Input: part model. Units: mm. Frame: model coordinates. Face numbers are marked on the shaded views. A direction names the side the tool comes from. Round coordinates to 2 decimals unless told otherwise and drop trailing zeros. Loops run counter-clockwise (first coordinate to the right, second up) from the corner with the lowest first, then second, coordinate; pieces in that order, holes last. Notation, with made-up numbers: (31, 51.5) - (42, 51.5) arc R35 ccw to (42, 89.5) - close; hole circle Ø9 at (44, 39). An arc over 180 degrees is marked (long way). One line per question, with ' | ' between items. Start each with the question number.
Item 1: Section D-D, the plane y = -21.25. Return loops of the section in (x, z), plus the area to 3 significant figures.
Item 2: Section A-A, the plane x = 6.5. Return loops of the section in (y, z), plus the area to 3 significant figures.
Item 3: Section B-B, the plane y = -8.75. Return loops of the section in (x, z).
Item 4: Material intervals for line 1 along Y through (x, z) = (26.5, 7); line 2 along X through (y, z) = (-4.25, 8.5); line 3 along X through (y, z) = (-1.5, 26), sorted ascending.
Item 5: First-contact query: pin 1 (19 mm diameter, centred on x = 9.5, z = 25.5, fed in from -Y). Flat tip, straight axial feed; report the tip coordinate or a pass-through.
Item 6: Section C-C, the plane z = 10.5. Return loops of the section in (x, y).
Item 7: Set-up query: the marked faces 1 and 2. Return all of +Z, -Z, +X, -X, +Y, -Y with unobstructed straight access to the full face (end or side cutting, diameter ignored); none if empty.
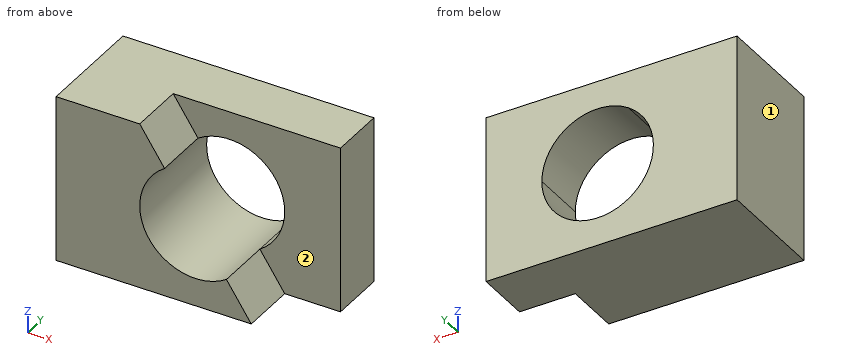
```python
from build123d import *

# Parameters (mm, degrees)
F0_W     = 57.15
F0_H     = 38.1
F1_DEPTH = 25.4
F2_W     = 12.7
F2_H     = 12.7
F3_DEPTH = 38.101
F5_DEPTH = 12.7
F7_DEPTH = 25.401


with BuildPart() as f1:
    # F0 (on Front) → F1 (new body)
    with BuildSketch(Plane.XZ):
        with Locations((0.037352, 19.05)):
            Rectangle(F0_W, F0_H)
    extrude(amount=F1_DEPTH)

    # F2 (on face) → F3 (cut, through all)
    with BuildSketch(Plane.XY.offset(38.1)):
        with Locations((22.262352, -19.05)):
            Rectangle(F2_W, F2_H)
    extrude(amount=-F3_DEPTH, mode=Mode.SUBTRACT)

    # F4 (on face) → F5 (cut)
    with BuildSketch(Plane.XZ.offset(25.4)):
        Polygon((15.912352, 38.1), (-9.487648, 38.1), (15.912352, 0), align=None)
    extrude(amount=-F5_DEPTH, mode=Mode.SUBTRACT)

    # F6 (on face) → F7 (cut, through all)
    with BuildSketch(Plane.XZ.offset(25.4)):
        with BuildLine():
            Line((10.257044, 8.482961), (-3.832341, 29.617039))
            ThreePointArc((-3.832341, 29.617039), (-7.354687, 12.005308), (10.257044, 8.482961))
        make_face()
        with BuildLine():
            ThreePointArc((10.257044, 8.482961), (14.409619, 13.057404), (15.912352, 19.05))
            ThreePointArc((15.912352, 19.05), (9.204947, 30.247267), (-3.832341, 29.617039))
            Line((-3.832341, 29.617039), (10.257044, 8.482961))
        make_face()
    extrude(amount=-F7_DEPTH, mode=Mode.SUBTRACT)


solid = f1.part
```
Return value:
1) outline: (-28.54, 0) - (15.91, 0) - (10.26, 8.48) arc R12.7 cw to (-3.83, 29.62) - (-9.49, 38.1) - (-28.54, 38.1) - close | area: 956 mm2
2) outline: (-25.4, 0) - (0, 0) - (0, 6.78) - (-25.4, 6.78) - close; (-12.7, 31.32) - (0, 31.32) - (0, 38.1) - (-12.7, 38.1) - close | area: 258 mm2
3) outline: (-28.54, 0) - (28.61, 0) - (28.61, 38.1) - (-28.54, 38.1) - close; hole (-3.83, 29.62) arc R12.7 ccw to (10.26, 8.48) arc R12.7 ccw to (15.91, 19.05) arc R12.7 ccw to start
4) line 1: -12.7 to 0 | line 2: -28.54 to -3.86, 10.28 to 28.61 | line 3: -28.54 to -7.42, 13.84 to 28.61
5) pin 1: y = -12.7
6) outline: (-28.54, -25.4) - (-6.18, -25.4) - (-6.18, 0) - (-28.54, 0) - close; (12.6, -12.7) - (28.61, -12.7) - (28.61, 0) - (12.6, 0) - close
7) face 1: +Z, -Z, -X, +Y, -Y | face 2: +Z, +X, -Y
